Source: CAD feature listing. Evaluate the final solid. Frame: model axes, mm. A direction names the side the tool comes from. Round coordinates to 2 decimals unless told otherwise and drop trailing zeros. Order: outer loops, then holes, each group sorted by start corner. A loop starts at its lowest first (then second) coordinate and runs counter-clockwise, first axis right, second up. Notation, with made-up numbers: M 56.5,85 L 75.5,85 A3 ccw 75.5,89 Z; hole C -13,76.25 d2. An arc over 180 degrees is marked long. Use one line per item in the form item = value. Start each with the question number.
Q1. Reachability of faces 1 (the flat face through (10.762, 8, 1)), 2 (the flat face through (11.972, 8, 1)) from +Z, -Z, +X, -X, +Y, -Y: full face, straight path, thin tool, end or side. Return the list, or none.
Q2. Contact query for a flat-ended pin moving along its axis: pin 1 (5 mm diameter, centred on x = 1, z = -23.5, fed in from +Y). Output: stop coordinate, or through.
Q3. Section A-A (y = 4.5). Return the cut outline in (x, z), plus the area to 3 significant figures.
Q4. Material intervals for probe 1 along X at (y, z) = (12.5, 54); probe 2 along Y at (x, z) = (-9.5, -39); probe 3 along X at (y, z) = (-0.3, 69.75), sorted ascending.
Q5. Section C-C (z = -34.5). Return the cut outline in (x, y), plus the area to 3 significant figures.
Q6. Section D-D (x = 5.5). Return the cut outline in (y, z), plus the area to 3 significant figures.
Q7. Section B-B (z = 36.75). Return the cut outline in (x, y).
Q8. Pull-direction query (Y, two-part tool) for faces 3 (the flat face through (-10.762, 8, -1)), 4 (the flat face through (0, 0, -1)), 5 (the cylindrical face through (-11.359, 9.27, -19.466)), 6 (the cylindrical face through (11.375, 9.27, -19.466)); classes: pulls with the +Y half, pulls with the -Y half, needs draft (parallel to the pull), parting line crosses it, or undercut.
from build123d import *

# Parameters (mm, degrees)
SKETCH1_W            = 20
SKETCH1_H            = 173.5
BASE_FLANGE1_DEPTH   = 1.21
EDGE_FLANGE1_DEPTH   = 173.5
EDGE_FLANGE2_DEPTH   = 173.5
SKETCH14_R           = 1.2
CUT_EXTRUDE1_DEPTH   = 5
M3_CLEARANCE_HOLE1_D = 3.4


# Sheet-metal steps are written as plain solids
with BuildPart() as part:
    # Sketch1 → Base-Flange1 (new body)
    with BuildSketch(Plane(origin=(0, 0, 0), x_dir=(1, 0, 0), z_dir=(0, 1, 0))):
        Rectangle(SKETCH1_W, SKETCH1_H)
    extrude(amount=-BASE_FLANGE1_DEPTH)

    # Edge-Flange1 section (across the edge) → Edge-Flange1 (add)
    with BuildSketch(Plane(origin=(-10.762, 0, -86.75), x_dir=(1, 0, 0), z_dir=(0, 0, 1))):
        with BuildLine():
            Line((-1.21, 0.762), (-1.21, 15))
            Line((-1.21, 15), (0, 15))
            Line((0, 15), (0, 0.762))
            ThreePointArc((0, 0.762), (0.223184633, 0.223184633), (0.762, 0))
            Line((0.762, 0), (0.762, -1.21))
            ThreePointArc((0.762, -1.21), (-0.632414572, -0.632414572), (-1.21, 0.762))
        make_face()
    extrude(amount=EDGE_FLANGE1_DEPTH)

    # Edge-Flange2 section (across the edge) → Edge-Flange2 (add)
    with BuildSketch(Plane(origin=(10.762, 0, 86.75), x_dir=(-1, 0, 0), z_dir=(0, 0, -1))):
        with BuildLine():
            Line((-1.21, 0.762), (-1.21, 15))
            Line((-1.21, 15), (0, 15))
            Line((0, 15), (0, 0.762))
            ThreePointArc((0, 0.762), (0.223184633, 0.223184633), (0.762, 0))
            Line((0.762, 0), (0.762, -1.21))
            ThreePointArc((0.762, -1.21), (-0.632414572, -0.632414572), (-1.21, 0.762))
        make_face()
    extrude(amount=EDGE_FLANGE2_DEPTH)

    # Sketch14 → Cut-Extrude1 (cut)
    with BuildSketch(Plane(origin=(0, -1.21, 0), x_dir=(-1, 0, 0), z_dir=(0, -1, 0))):
        with Locations(Location((0, -69.75, 0), (0, 0, 90))):
            Circle(SKETCH14_R)
    extrude(amount=-CUT_EXTRUDE1_DEPTH, mode=Mode.SUBTRACT)

    # M3 Clearance Hole1 (through all)
    with Locations(Plane(origin=(-11.972, 85.70162808, 15.202320986), x_dir=(0, 0, -1), z_dir=(-1, 0, 0))):
        with Locations((-21.547679014, 77.93962808), (35.452320986, 77.93962808)):
            Hole(M3_CLEARANCE_HOLE1_D / 2)


solid = part.part
Results list:
q1.face_1 = +Z, -Z, +Y
q1.face_2 = +Z, -Z, +X, +Y, -Y
q2.pin_1 = 0
q3.outline = M -11.97,-86.75 L -10.76,-86.75 L -10.76,86.75 L -11.97,86.75 Z; M 10.76,-86.75 L 11.97,-86.75 L 11.97,86.75 L 10.76,86.75 Z
q3.area = 420 mm2
q4.probe_1 = -11.97 to -10.76, 10.76 to 11.97
q4.probe_2 = -1.21 to 0
q4.probe_3 = -11.66 to -1.2, 1.2 to 11.66
q5.outline = M -11.97,0.76 A1.97 ccw -10,-1.21 L 10,-1.21 A1.97 ccw 11.97,0.76 L 11.97,15 L 10.76,15 L 10.76,0.76 A0.76 cw 10,0 L -10,0 A0.76 cw -10.76,0.76 L -10.76,15 L -11.97,15 Z
q5.area = 63.9 mm2
q6.outline = M -1.21,-86.75 L 0,-86.75 L 0,86.75 L -1.21,86.75 Z
q6.area = 210 mm2
q7.outline = M -11.97,0.76 A1.97 ccw -10,-1.21 L 10,-1.21 A1.97 ccw 11.97,0.76 L 11.97,6.06 L 10.76,6.06 L 10.76,0.76 A0.76 cw 10,0 L -10,0 A0.76 cw -10.76,0.76 L -10.76,6.06 L -11.97,6.06 Z; M -11.97,9.46 L -10.76,9.46 L -10.76,15 L -11.97,15 Z; M 10.76,9.46 L 11.97,9.46 L 11.97,15 L 10.76,15 Z
q8.face_3 = needs draft
q8.face_4 = pulls with the +Y half
q8.face_5 = undercut
q8.face_6 = undercut
